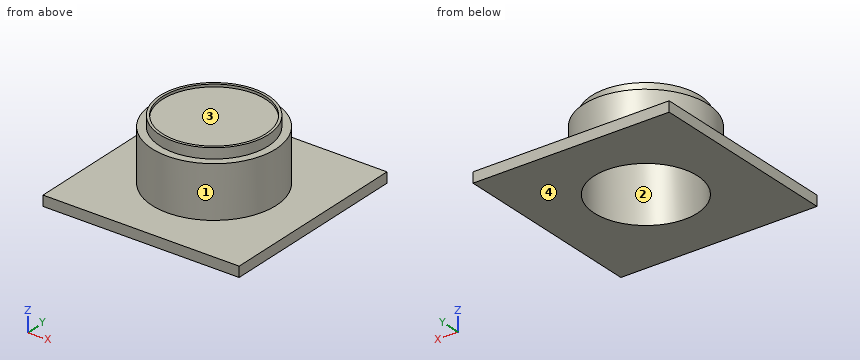
from build123d import *

# Parameters (mm, degrees)
SKETCH1_W           = 19
SKETCH1_H           = 19
BOSS_EXTRUDE1_DEPTH = 1
SKETCH2_R           = 6
BOSS_EXTRUDE2_DEPTH = 5
SKETCH3_R           = 5.25
SKETCH3_R_2         = 5
BOSS_EXTRUDE5_DEPTH = 1
SKETCH6_R           = 5
CUT_EXTRUDE3_DEPTH  = 16.203073736
SKETCH7_R           = 5.25
BOSS_EXTRUDE6_DEPTH = 0.75


with BuildPart() as part:
    # Sketch1 → Boss-Extrude1 (new body)
    with BuildSketch(Plane.XY):
        with Locations((0.085585586, 0)):
            Rectangle(SKETCH1_W, SKETCH1_H)
    extrude(amount=BOSS_EXTRUDE1_DEPTH)

    # Sketch2 → Boss-Extrude2 (add)
    with BuildSketch(Plane.XY.offset(1)):
        Circle(SKETCH2_R)
    extrude(amount=BOSS_EXTRUDE2_DEPTH)

    # Sketch3 → Boss-Extrude5 (add)
    with BuildSketch(Plane.XY.offset(6)):
        Circle(SKETCH3_R)
        Circle(SKETCH3_R_2, mode=Mode.SUBTRACT)
    extrude(amount=BOSS_EXTRUDE5_DEPTH)

    # Sketch6 → Cut-Extrude3 (cut, through all)
    with BuildSketch(Plane.XY.offset(7)):
        Circle(SKETCH6_R)
    extrude(amount=-CUT_EXTRUDE3_DEPTH, mode=Mode.SUBTRACT)

    # Sketch7 → Boss-Extrude6 (add)
    with BuildSketch(Plane.XY.offset(6)):
        Circle(SKETCH7_R)
    extrude(amount=BOSS_EXTRUDE6_DEPTH)


solid = part.part
Source: CAD feature listing. Evaluate the final solid. Frame: model axes, mm. Face numbers are marked on the shaded views. Round coordinates to 2 decimals unless told otherwise and drop trailing zeros. Loops run counter-clockwise (first coordinate to the right, second up) from the corner with the lowest first, then second, coordinate; pieces in that order, holes last. Notation, with made-up numbers: (23, -20.5) -> (36, -20.5) arc R8 cw to (36, -6.5) -> close; hole circle Ø4 at (34.5, 49.25). An arc over 180 degrees is marked (long way). Answer as a JSON object with one key per item and string values. Group by question number.
Q1. Ray query, line 1 (Y direction, x = 0, z = 4.05); line 2 (Y direction, x = 0, z = 6.9); line 3 (Z direction, x = 3.5, y = 8.5). Return the intervals inside material, ascending. Write a range as from..to.
Q2. Mould query, pull axis X, two halves, no side actions, for the marked faces 1, 2, 3 and 4. Classes: pulls with the +X half, pulls with the -X half, needs draft (parallel to the pull), parting line crosses it, or undercut.
Q3. Section query D-D (x = 7.5). Output: boundary loops of the cut face in (y, z), plus the area to 3 significant figures.
Q4. Section query C-C (z = 4.5). Output: boundary loops of the cut face in (x, y).
Q5. Section query B-B (y = 0). Output: boundary loops of the cut face in (x, z).
Q6. Section query A-A (x = 0). Output: boundary loops of the cut face in (y, z), plus the area to 3 significant figures.
Q7. Contact query for flat-ended pins moving along their axis: P1, Ø3, axis at x = 2.5, y = -0.5, coming from the +Z side; P2, Ø1.5, axis at y = -2.5, z = 3, coming from the -X side. Output: stop coordinate, or through.
Completed:
{
 "1": {"line 1": "-6..-5, 5..6", "line 2": "-5.25..-5, 5..5.25", "line 3": "0..1"},
 "2": {"face 1": "parting line crosses it", "face 2": "undercut", "face 3": "undercut", "face 4": "needs draft"},
 "3": {"outline": "(-9.5, 0) -> (9.5, 0) -> (9.5, 1) -> (-9.5, 1) -> close", "area": "19.0 mm²"},
 "4": {"outline": "circle Ø12 at (0, 0); hole circle Ø10 at (0, 0)"},
 "5": {"outline": "(-9.41, 0) -> (-5, 0) -> (-5, 6) -> (5, 6) -> (5, 0) -> (9.59, 0) -> (9.59, 1) -> (6, 1) -> (6, 6) -> (5.25, 6) -> (5.25, 7) -> (5, 7) -> (5, 6.75) -> (-5, 6.75) -> (-5, 7) -> (-5.25, 7) -> (-5.25, 6) -> (-6, 6) -> (-6, 1) -> (-9.41, 1) -> close"},
 "6": {"outline": "(-9.5, 0) -> (-5, 0) -> (-5, 6) -> (5, 6) -> (5, 0) -> (9.5, 0) -> (9.5, 1) -> (6, 1) -> (6, 6) -> (5.25, 6) -> (5.25, 7) -> (5, 7) -> (5, 6.75) -> (-5, 6.75) -> (-5, 7) -> (-5.25, 7) -> (-5.25, 6) -> (-6, 6) -> (-6, 1) -> (-9.5, 1) -> close", "area": "27.0 mm²"},
 "7": {"P1": "z = 6.75", "P2": "x = -5.74"}
}
